from build123d import *

# Parameters (mm, degrees)
SKETCH1_R           = 37
BOSS_EXTRUDE1_DEPTH = 5
CUT_EXTRUDE3_START  = -10
CUT_EXTRUDE3_DEPTH  = 10
FILLET1_R           = 25
FILLET2_R           = 20
SKETCH11_W          = 7
SKETCH11_H          = 5
CUT_EXTRUDE4_DEPTH  = 10
SKETCH12_W          = 10
SKETCH12_H          = 7
CUT_EXTRUDE5_DEPTH  = 10


with BuildPart() as part:
    # Sketch1 → Boss-Extrude1 (new body)
    with BuildSketch(Plane.XY):
        Circle(SKETCH1_R)
    extrude(amount=BOSS_EXTRUDE1_DEPTH)

    # Sketch10 → Cut-Extrude3 (cut)
    with BuildSketch(Plane.XY.offset(5).offset(CUT_EXTRUDE3_START)):
        with BuildLine():
            Line((-25, 27.276363394), (-25, -27.276363394))
            ThreePointArc((-25, -27.276363394), (-37, 0), (-25, 27.276363394))
        make_face()
        with BuildLine():
            Line((25, -27.276363394), (25, 27.276363394))
            ThreePointArc((25, 27.276363394), (37, 0), (25, -27.276363394))
        make_face()
    extrude(amount=CUT_EXTRUDE3_DEPTH, mode=Mode.SUBTRACT)

    # Fillet1
    fillet1_edges = [part.edges().sort_by_distance(p)[0] for p in [
        (-25, 27.276363394, 2.5),
        (25, 27.276363394, 2.5),
    ]]
    fillet(fillet1_edges, radius=FILLET1_R - 0.0001)  # a hair under: the kernel refuses the full size

    # Fillet2
    fillet2_edges = [part.edges().sort_by_distance(p)[0] for p in [
        (-25, -27.276363394, 2.5),
        (25, -27.276363394, 2.5),
    ]]
    fillet(fillet2_edges, radius=FILLET2_R)

    # Sketch11 → Cut-Extrude4 (cut)
    with BuildSketch(Plane.XY.offset(5)):
        with Locations((0, 2)):
            Rectangle(SKETCH11_W, SKETCH11_H)
        with Locations((0, -18)):
            Rectangle(SKETCH11_W, SKETCH11_H)
    extrude(amount=-CUT_EXTRUDE4_DEPTH, mode=Mode.SUBTRACT)

    # Sketch12 → Cut-Extrude5 (cut)
    with BuildSketch(Plane.XY.offset(5)):
        with Locations((13, -9)):
            Rectangle(SKETCH12_W, SKETCH12_H)
    extrude(amount=-CUT_EXTRUDE5_DEPTH, mode=Mode.SUBTRACT)


solid = part.part
Geometry check sheet. Reference: the model listing, model coordinates, mm. A direction names the side the tool comes from. Give positions to 0.01 mm unless a question says otherwise; leave off trailing zeros. Order: outer loops, then holes, each group sorted by start corner. A loop starts at its lowest first (then second) coordinate and runs counter-clockwise, first axis right, second up. Notation, with made-up numbers: (39, 71.25) - (71, 71.25) arc R27 cw to (71, 91.25) - close; hole circle Ø11 at (46.25, 41). An arc over 180 degrees is marked (long way). Answer as a JSON object with one key per item and string values.
(1) Tool access check on faces 1 (the cylindrical face through (21.19, -27.99, 2.54)), 2 (the flat face through (3.5, 2, 3)). Record the directions out of +Z, -Z, +X, -X, +Y, -Y that give a thin tool (end or side, any length) a straight path to the whole face; none if there is none.
Report:
{"face 1": "+Z, -Z, +X, -Y", "face 2": "+Z, -Z"}
(2) Cross-section at D-D (x = -2.5). Record the cut outline in (y, z), then the cut area to 3 significant figures.
Report:
{"outline": "(-36.92, 0) - (-20.5, 0) - (-20.5, 5) - (-36.92, 5) - close; (-15.5, 0) - (-0.5, 0) - (-0.5, 5) - (-15.5, 5) - close; (4.5, 0) - (36.87, 0) - (36.87, 5) - (4.5, 5) - close", "area": "319 mm^2"}
(3) Draft check along Y on faces 3 (the flat face through (-3.5, 2, 3)), 4 (the cylindrical face through (-17.482, 29.871, 2.535)), 5 (the flat face through (-25, -2, 2)). Enter one of: released by +Y, released by -Y, zero draft, split by the parting line, or undercut.
Report:
{"face 3": "undercut", "face 4": "released by +Y", "face 5": "zero draft"}
(4) Material ranges on line 1 (X direction, y = -10, z = 1.35); line 2 (Y direction, x = 1, z = 1.9); line 3 (X direction, y = 1, z = 0.3), recorded low to high.
Report:
{"line 1": "-25 to 8, 18 to 25", "line 2": "-36.99 to -20.5, -15.5 to -0.5, 4.5 to 36.98", "line 3": "-25 to -3.5, 3.5 to 25"}
(5) Cross-section at C-C (x = 9). Record the cut outline in (y, z), then the cut area to 3 significant figures.
Report:
{"outline": "(-35.89, 0) - (-12.5, 0) - (-12.5, 5) - (-35.89, 5) - close; (-5.5, 0) - (35.32, 0) - (35.32, 5) - (-5.5, 5) - close", "area": "321 mm^2"}
(6) Cross-section at A-A (y = -8). Record the cut outline in (x, z).
Report:
{"outline": "(-25, 0) - (8, 0) - (8, 5) - (-25, 5) - close; (18, 0) - (25, 0) - (25, 5) - (18, 5) - close"}
(7) Depth check by flat-ended pin: pin 1 Ø3 at (y, z) = (16, 0.5) entering from -X; pin 2 Ø5 at (x, y) = (9, -6) entering from +Z; pin 3 Ø1.5 at (x, z) = (15.5, 3.5) entering from +Y; pin 4 Ø1.5 at (x, z) = (-1, 3.5) entering from -Y. Enter the tip coordinate at first touch or a pass-through.
Report:
{"pin 1": "x = -24.87", "pin 2": "z = 5", "pin 3": "y = 32.19", "pin 4": "y = -37"}
(8) Cross-section at B-B (z = 0.85). State how many separate pieces and enclosed holes the cut face has, then the cut area to 3 significant figures.
Report:
{"separate pieces": "1", "enclosed holes": "3", "area": "3,090 mm^2"}
